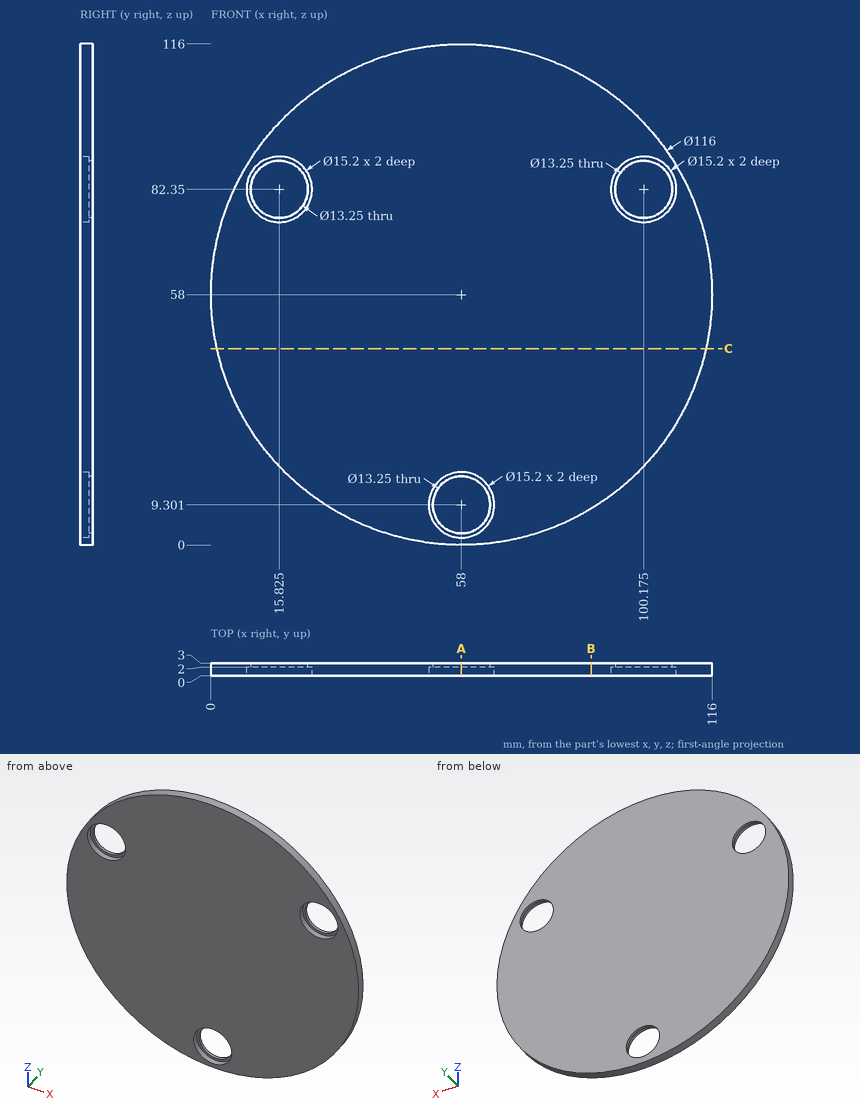
Could you check a few things on this drawing? It's one solid part, dimensions in mm from its lowest x, y, z. Coordinates: 2 decimals unless noted, no trailing zeros. Order: outer loops, then holes, each group sorted by start corner. A loop starts at its lowest first (then second) coordinate and runs counter-clockwise, first axis right, second up. Notation, with made-up numbers: (38, 61) -> (93, 61) arc R9 ccw to (93, 76) -> close; hole circle Ø3 at (55, 19). An arc over 180 degrees is marked (long way). Answer in a Markdown table with one row per item.
(1) Please list where these lines run through material, in increasing order: probe 1 along Z at (x, y) = (58, 0.7); probe 2 along Z at (x, y) = (58, 2.45) (1 decimal); probe 3 along X at (y, z) = (2.65, 77) (1 decimal).
Answer key:
| item | result |
|---|---|
| probe 1 | 0 to 1.7, 16.9 to 116 |
| probe 2 | 0 to 2.7, 15.9 to 116 |
| probe 3 | 3.2 to 11.9, 19.7 to 96.3, 104.1 to 112.8 |
(2) I want a section at B-B on x = 88. List the corners of the cut face in (y, z) for me.
Answer key:
| item | result |
|---|---|
| outline | (0, 8.36) -> (3, 8.36) -> (3, 107.64) -> (0, 107.64) -> close |
(3) Will these pins go through, and if not, where does the flat tip stop? pin 1 Ø1.5 at (x, y) = (51, 1) entering from +Z; pin 2 Ø4.5 at (x, z) = (56, 7.5) entering from -Y; pin 3 Ø1.5 at (x, y) = (32.5, 1) entering from -Z (1 decimal); pin 4 Ø7.5 at (x, z) = (98.5, 85.5) entering from -Y.
Answer key:
| item | result |
|---|---|
| pin 1 | z = 115.66 |
| pin 2 | through |
| pin 3 | z = 5.5 |
| pin 4 | y = 2 |
(4) I want a section at A-A on x = 58. List the corners of the cut face in (y, z) for me (1 decimal).
Answer key:
| item | result |
|---|---|
| outline | (0, 0) -> (3, 0) -> (3, 2.7) -> (2, 2.7) -> (2, 1.7) -> (0, 1.7) -> close; (0, 16.9) -> (2, 16.9) -> (2, 15.9) -> (3, 15.9) -> (3, 116) -> (0, 116) -> close |
(5) I want a section at C-C on z = 45.5. List the corners of the cut face in (x, y) for me.
Answer key:
| item | result |
|---|---|
| outline | (1.36, 0) -> (114.64, 0) -> (114.64, 3) -> (1.36, 3) -> close |
